from build123d import *

# Parameters (mm, degrees)
SKETCH1_R          = 31.75
SKETCH1_R_2        = 5.5626
EXTRUDE1_DEPTH     = 3.175
CUT_EXTRUDE1_DEPTH = 4.175


with BuildPart() as part:
    # Sketch1 → Extrude1 (new body)
    with BuildSketch(Plane.XY):
        Circle(SKETCH1_R)
        with Locations((0, 23.78973844)):
            Circle(SKETCH1_R_2, mode=Mode.SUBTRACT)
        with Locations((20.602517839, 11.89486922)):
            Circle(SKETCH1_R_2, mode=Mode.SUBTRACT)
        with Locations((20.602517839, -11.89486922)):
            Circle(SKETCH1_R_2, mode=Mode.SUBTRACT)
        with Locations((0, -23.78973844)):
            Circle(SKETCH1_R_2, mode=Mode.SUBTRACT)
        with Locations((-20.602517839, -11.89486922)):
            Circle(SKETCH1_R_2, mode=Mode.SUBTRACT)
        with Locations((-20.602517839, 11.89486922)):
            Circle(SKETCH1_R_2, mode=Mode.SUBTRACT)
    extrude(amount=EXTRUDE1_DEPTH)

    # Sketch2 → Cut-Extrude1 (cut, through all)
    with BuildSketch(Plane(origin=(0, 0, 0), x_dir=(-1, 0, 0), z_dir=(0, 0, -1))):
        with BuildLine():
            Line((8.878771943, 21.061731462), (8.878771943, 30.483272606))
            ThreePointArc((8.878771943, 30.483272606), (15.875, 27.49630657), (21.959902496, 22.93087836))
            Line((21.959902496, 22.93087836), (13.800608523, 18.220107788))
            ThreePointArc((13.800608523, 18.220107788), (11.42835425, 19.794490207), (8.878771943, 21.061731462))
        make_face()
        with BuildLine():
            Line((-8.878771943, 30.483272606), (-8.878771943, 21.061731462))
            ThreePointArc((-8.878771943, 21.061731462), (-11.42835425, 19.794490207), (-13.800608523, 18.220107788))
            Line((-13.800608523, 18.220107788), (-21.959902496, 22.93087836))
            ThreePointArc((-21.959902496, 22.93087836), (-15.875, 27.49630657), (-8.878771943, 30.483272606))
        make_face()
        with BuildLine():
            Line((22.679380466, 2.841623674), (30.838674439, 7.552394246))
            ThreePointArc((30.838674439, 7.552394246), (31.75, 0), (30.838674439, -7.552394246))
            Line((30.838674439, -7.552394246), (22.679380466, -2.841623674))
            ThreePointArc((22.679380466, -2.841623674), (22.856708499, 0), (22.679380466, 2.841623674))
        make_face()
        with BuildLine():
            Line((13.800608523, -18.220107788), (21.959902496, -22.93087836))
            ThreePointArc((21.959902496, -22.93087836), (15.875, -27.49630657), (8.878771943, -30.483272606))
            Line((8.878771943, -30.483272606), (8.878771943, -21.061731462))
            ThreePointArc((8.878771943, -21.061731462), (11.42835425, -19.794490207), (13.800608523, -18.220107788))
        make_face()
        with BuildLine():
            Line((-8.878771943, -21.061731462), (-8.878771943, -30.483272606))
            ThreePointArc((-8.878771943, -30.483272606), (-15.875, -27.49630657), (-21.959902496, -22.93087836))
            Line((-21.959902496, -22.93087836), (-13.800608523, -18.220107788))
            ThreePointArc((-13.800608523, -18.220107788), (-11.42835425, -19.794490207), (-8.878771943, -21.061731462))
        make_face()
        with BuildLine():
            Line((-22.679380466, -2.841623674), (-30.838674439, -7.552394246))
            ThreePointArc((-30.838674439, -7.552394246), (-31.75, 0), (-30.838674439, 7.552394246))
            Line((-30.838674439, 7.552394246), (-22.679380466, 2.841623674))
            ThreePointArc((-22.679380466, 2.841623674), (-22.856708499, 0), (-22.679380466, -2.841623674))
        make_face()
    extrude(amount=-CUT_EXTRUDE1_DEPTH, mode=Mode.SUBTRACT)


solid = part.part
For this review, take the finished solid that the model builds, in its own axes (mm). A direction names the side the tool comes from. Coordinates: 2 decimals unless noted, no trailing zeros. Loops run counter-clockwise (first coordinate to the right, second up) from the corner with the lowest first, then second, coordinate; pieces in that order, holes last. Notation, with made-up numbers: (35.5, 39.5) - (88.5, 39.5) arc R24 cw to (88.5, 52.5) - close; hole circle Ø7 at (-19.75, 86.5). An arc over 180 degrees is marked (long way). Return JSON: item names as keys, results as strings.
Item 1: Insertion check: pin 1 (14.5 mm diameter, centred on x = -20.6, y = 11.89, fed in from -Z); pin 2 (1 mm diameter, centred on y = -28, z = 1, fed in from +X); pin 3 (1.5 mm diameter, centred on x = -19.5, z = 1, fed in from -Y); pin 4 (1 mm diameter, centred on y = -24.5, z = 2, fed in from -X). Each pin has a flat end and moves straight along its axis. Give the tip position at first contact, or say it passes through.
Determined:
{"pin 1": "stops at z = 0", "pin 2": "stops at x = 8.88", "pin 3": "stops at y = -21.94", "pin 4": "stops at x = -8.88"}
Item 2: Mouldability with a two-part tool opening along X and no side actions: class faces 5 (the flat face through (-26.82, -5.23, 1.57)), 6 (the flat face through (0, 0, 3.175)), 7 (the flat face through (-17.94, 20.61, 1.57)), 8 (the cylindrical face through (22.857, 0.04, 1.565)) as pulls with the +X half, pulls with the -X half, needs draft (parallel to the pull), parting line crosses it, or undercut.
Determined:
{"face 5": "pulls with the -X half", "face 6": "needs draft", "face 7": "undercut", "face 8": "pulls with the +X half"}
Item 3: For line 1 (Y direction, x = 0, z = 2.15); line 2 (X direction, y = 24, z = 1.3); line 3 (Y direction, x = -20, z = 2.65) (3 decimals), list the stretches that pass through material, from the lowest coordinate up.
Determined:
{"line 1": "y = -31.75 to -29.35, -18.23 to 18.23, 29.35 to 31.75", "line 2": "x = -8.88 to -5.56, 5.56 to 8.88", "line 3": "y = -21.799 to -17.425, -6.365 to 6.365, 17.425 to 21.799"}
Item 4: Take a section at B-B (z = 2.2). State how many separate pieces and enclosed holes the cut face has, then the cut area to 3 significant figures.
Determined:
{"separate pieces": "1", "enclosed holes": "6", "area": "2,020 mm2"}
Item 5: For faces 1 (the flat face through (-8.879, -26, 2)), 2 (the flat face through (17.82, 20.54, 1.57)), 3 (the cylindrical face through (-1.21, 18.36, 1.57)), 4 (the flat face through (26.702, -5.164, 1.565)), list the 3-axis set-ups (+Z, -Z, +X, -X, +Y, -Y) from which the entire face can be reached by the end or side of a thin tool; tool diameter is ignored.
Determined:
{"face 1": "+Z, -Z, -Y", "face 2": "+Z, -Z, +Y", "face 3": "+Z, -Z", "face 4": "+Z, -Z, +X"}
Item 6: Take a section at A-A (x = 0). Give the boundary of the cut face in (y, z) (3 decimals).
Determined:
{"outline": "(-31.75, 0) - (-29.352, 0) - (-29.352, 3.175) - (-31.75, 3.175) - close; (-18.227, 0) - (18.227, 0) - (18.227, 3.175) - (-18.227, 3.175) - close; (29.352, 0) - (31.75, 0) - (31.75, 3.175) - (29.352, 3.175) - close"}
Item 7: Take a section at C-C (y = -14). Give the boundary of the cut face in (x, z) (3 decimals).
Determined:
{"outline": "(-28.497, 0) - (-25.751, 0) - (-25.751, 3.175) - (-28.497, 3.175) - close; (-15.454, 0) - (15.454, 0) - (15.454, 3.175) - (-15.454, 3.175) - close; (25.751, 0) - (28.497, 0) - (28.497, 3.175) - (25.751, 3.175) - close"}
Item 8: Take a section at D-D (x = 27.5). Give the boundary of the cut face in (y, z) (3 decimals), then the cut area to 3 significant figures.
Determined:
{"outline": "(-15.869, 0) - (-5.625, 0) - (-5.625, 3.175) - (-15.869, 3.175) - close; (5.625, 0) - (15.869, 0) - (15.869, 3.175) - (5.625, 3.175) - close", "area": "65.0 mm2"}
